Can you work these out from the model? Positions are in its coordinate system, mm. Give positions to 0.01 mm unless a question says otherwise; leave off trailing zeros. Loops run counter-clockwise (first coordinate to the right, second up) from the corner with the lowest first, then second, coordinate; pieces in that order, holes last.
from build123d import *

# Parameters (mm, degrees)
F1_DEPTH      = 920
F2_W          = 32.354593277
F2_H          = 26.2916557118
F3_DEPTH      = 25
F3_DEPTH_BACK = 25
F4_W          = 93.2869557291
F4_H          = 71.5390760452
F5_DEPTH      = 3
F5_DEPTH_BACK = 25


with BuildPart() as f1:
    # F0 (on Top) → F1 (new body)
    with BuildSketch(Plane.XY):
        with BuildLine():
            Line((29.9719494759, 0.0280495928), (-0.0280505241, 0.0280495928))
            Line((-0.0280505241, 0.0280495928), (-0.0280505241, -29.9719504072))
            Line((-0.0280505241, -29.9719504072), (1.9719494759, -29.9719504072))
            ThreePointArc((1.9719494759, -29.9719504072), (2.679056257, -29.6790571884), (2.9719494759, -28.9719504072))
            Line((2.9719494759, -28.9719504072), (2.9719494759, -3.9719504072))
            ThreePointArc((2.9719494759, -3.9719504072), (3.2648426947, -3.264843626), (3.9719494759, -2.9719504072))
            Line((3.9719494759, -2.9719504072), (28.9719494759, -2.9719504072))
            ThreePointArc((28.9719494759, -2.9719504072), (29.679056257, -2.6790571884), (29.9719494759, -1.9719504072))
            Line((29.9719494759, -1.9719504072), (29.9719494759, 0.0280495928))
        make_face()
    extrude(amount=F1_DEPTH)

    # F2 (on Front) → F3 (cut, two sides)
    with BuildSketch(Plane.XZ) as f3_sk:
        with Locations((19.1772966385, 1.8541721441)):
            Rectangle(F2_W, F2_H)
        with Locations((19.1772966385, 918.1458278559)):
            Rectangle(F2_W, F2_H)
    extrude(amount=F3_DEPTH, mode=Mode.SUBTRACT)
    extrude(f3_sk.sketch, amount=-F3_DEPTH_BACK, mode=Mode.SUBTRACT)

    # F4 (on Right) → F5 (cut, two sides)
    with BuildSketch(Plane.YZ) as f5_sk:
        with Locations((-15.7623803243, -5.7695380226)):
            Rectangle(F4_W, F4_H)
        with Locations((-15.7623803243, 925.7695380226)):
            Rectangle(F4_W, F4_H)
    extrude(amount=F5_DEPTH, mode=Mode.SUBTRACT)
    extrude(f5_sk.sketch, amount=-F5_DEPTH_BACK, mode=Mode.SUBTRACT)


solid = f1.part
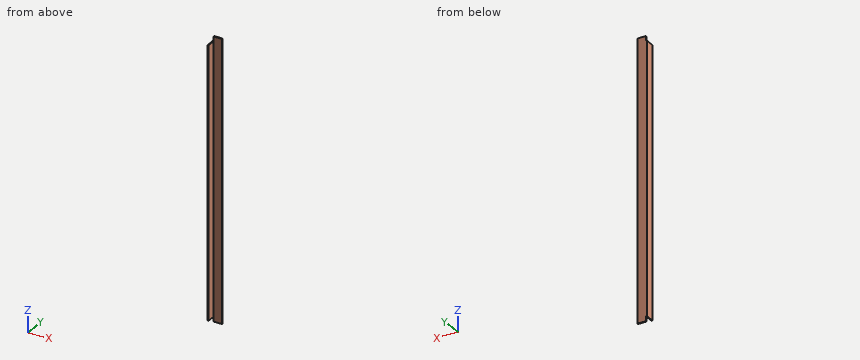
(1) Will these pins go through, and if not, where does the flat tip stop? P1, Ø12.5, axis at y = -17, z = 377.5, coming from the +X side; P2, Ø4, axis at x = 4, y = -3.5, coming from the -Z side; P3, Ø4, axis at y = -2.5, z = 895.5, coming from the -X side; P4, Ø3.5, axis at x = 1.5, y = -12.5, coming from the +Z side.
Returned:
P1: stops at x = 2.97
P2: stops at z = 15
P3: stops at x = 3
P4: stops at z = 890
(2) Please list where these lines run through material, in increasing order: probe 1 along Y at (x, z) = (7.5, 59); probe 2 along X at (y, z) = (-24, 259); probe 3 along X at (y, z) = (-2.5, 673).
Returned:
probe 1: y = -2.97 to 0.03
probe 2: x = -0.03 to 2.97
probe 3: x = -0.03 to 29.82
(3) Suppose I cut it at C-C on x = 8.75. List the corners of the cut face in (y, z) for me.
Returned:
outline: (-2.97, 15) - (0.03, 15) - (0.03, 905) - (-2.97, 905) - close
(4) Suppose I cut it at B-B on y = -10.5. List the corners of the cut face in (x, z) for me.
Returned:
outline: (-0.03, 30) - (2.97, 30) - (2.97, 890) - (-0.03, 890) - close
(5) Suppose I cut it at A-A on z = 259.5. List the corners of the cut face in (x, y) for me.
Returned:
outline: (-0.03, -29.97) - (1.97, -29.97) arc R1 ccw to (2.97, -28.97) - (2.97, -3.97) arc R1 cw to (3.97, -2.97) - (28.97, -2.97) arc R1 ccw to (29.97, -1.97) - (29.97, 0.03) - (-0.03, 0.03) - close
